For this review, take the finished solid that the model builds, in its own axes (mm). Face numbers are marked on the shaded views. A direction names the side the tool comes from. Round coordinates to 2 decimals unless told otherwise and drop trailing zeros. Write each loop counter-clockwise with the first axis right and the second up, starting at its lowest first coordinate (ties: lowest second). Pieces come first, ordered by that corner, then holes. Notation, with made-up numbers: M 69.25,70.5 L 79.25,70.5 A30 cw 79.25,93.5 Z; hole C 85,72 d3. An arc over 180 degrees is marked long. One line per question, with ' | ' between items.
```python
from build123d import *

# Parameters (mm, degrees)
SKETCH1_R               = 11
SKETCH1_R_2             = 2.669858215
BOSS_EXTRUDE1_DEPTH     = 2
SKETCH2_R               = 4.05
BOSS_EXTRUDE2_DEPTH     = 3
SKETCH3_R               = 4
SKETCH3_R_2             = 2.669858215
BOSS_EXTRUDE3_DEPTH     = 1
CHAMFER1_SIZE           = 0.6
M2_TAPPED_HOLE1_D       = 1.6
M2_5_TAPPED_HOLE1_D     = 2.05
M2_5_TAPPED_HOLE1_DEPTH = 6.35
M2_5_TAPPED_HOLE1_TIP   = 0.615882135


with BuildPart() as part:
    # Sketch1 → Boss-Extrude1 (new body)
    with BuildSketch(Plane.XY):
        Circle(SKETCH1_R)
        Circle(SKETCH1_R_2, mode=Mode.SUBTRACT)
    extrude(amount=BOSS_EXTRUDE1_DEPTH)

    # Sketch2 → Boss-Extrude2 (add)
    with BuildSketch(Plane.XY.offset(2)):
        Circle(SKETCH2_R)
    extrude(amount=BOSS_EXTRUDE2_DEPTH)

    # Sketch3 → Boss-Extrude3 (add)
    with BuildSketch(Plane(origin=(0, 0, 0), x_dir=(-1, 0, 0), z_dir=(0, 0, -1))):
        Circle(SKETCH3_R)
        Circle(SKETCH3_R_2, mode=Mode.SUBTRACT)
    extrude(amount=BOSS_EXTRUDE3_DEPTH)

    # Chamfer1
    chamfer1_edges = [part.edges().sort_by_distance(p)[0] for p in [
        (4, 0, -1),
    ]]
    chamfer(chamfer1_edges, length=CHAMFER1_SIZE)

    # M2 Tapped Hole1 (through all)
    with Locations(Plane.XY.offset(2)):
        with Locations((2.286188648, 7.666377336), (7.037526898, 3.804367906), (7.666377336, -2.286188648), (3.804367906, -7.037526898), (-2.286188648, -7.666377336), (-7.037526898, -3.804367906), (-7.666377336, 2.286188648), (-3.804367906, 7.037526898)):
            Hole(M2_TAPPED_HOLE1_D / 2)

    # M2.5 Tapped Hole1
    with Locations(Plane.XY.offset(5)):
        with Locations((0, 0)):
            Hole(M2_5_TAPPED_HOLE1_D / 2, depth=M2_5_TAPPED_HOLE1_DEPTH)
            with Locations((0, 0, -(M2_5_TAPPED_HOLE1_DEPTH + M2_5_TAPPED_HOLE1_TIP / 2))):  # 118° drill point
                Cone(0, M2_5_TAPPED_HOLE1_D / 2, M2_5_TAPPED_HOLE1_TIP, mode=Mode.SUBTRACT)


solid = part.part
```
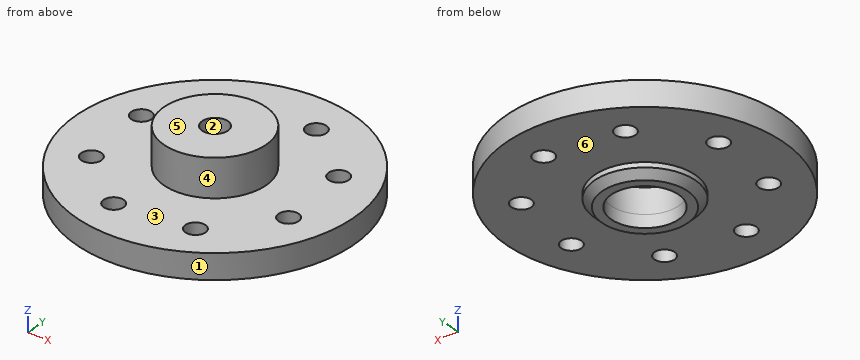
Item 1: Machinability: for the marked faces 4, 5 and 6, which of the approach directions +Z, -Z, +X, -X, +Y, -Y give a long, thin tool a straight path to every point of the face, cutting with its end or side? Answer none if there is none.
Results:
face 4: +Z | face 5: +Z, +X, -X, +Y, -Y | face 6: -Z
Item 2: Take a section at C-C (z = 1.4). State how many separate pieces and enclosed holes the cut face has, then the cut area to 3 significant figures.
Results:
separate pieces: 1 | enclosed holes: 9 | area: 342 mm2
Item 3: To check wall thickness, follow line 1 along Y through (x, z) = (1.75, 1.9); line 2 along Y through (x, z) = (0, 4.35) (3 decimals); line 3 along Z through (x, y) = (0, 7.5). State the ranges of each line that lie inside material, in increasing order. Write a range as from..to.
Results:
line 1: -10.86..-2.02, 2.02..7.07, 8.26..10.86 | line 2: -4.05..-1.025, 1.025..4.05 | line 3: 0..2
Item 4: Insertion check: pin 1 Ø5 at (x, y) = (0, 0) entering from -Z; pin 2 Ø1.8 at (x, y) = (-3.8, 7.04) entering from +Z; pin 3 Ø1.3 at (x, y) = (-2.29, -7.67) entering from +Z; pin 4 Ø1.5 at (y, z) = (-7, 1) entering from -X. Each pin has a flat end and moves straight along its axis. Give the tip position at first contact, or say it passes through.
Results:
pin 1: z = 2 | pin 2: z = 2 | pin 3: through | pin 4: x = -9.05
Item 5: Take a section at A-A (x = 0). Write out the cut boundary in (y, z) (3 decimals).
Results:
outline: M -11,0 L -4,0 L -4,-0.4 L -3.4,-1 L -2.67,-1 L -2.67,2 L -1.025,2 L -1.025,5 L -4.05,5 L -4.05,2 L -11,2 Z; M 1.025,2 L 2.67,2 L 2.67,-1 L 3.4,-1 L 4,-0.4 L 4,0 L 11,0 L 11,2 L 4.05,2 L 4.05,5 L 1.025,5 Z
Item 6: Mouldability with a two-part tool opening along X and no side actions: class the marked faces 1, 2 and 3 as +X half, -X half, draft (parallel to the pull), parting line (faces both ways), or undercut.
Results:
face 1: parting line | face 2: undercut | face 3: draft
Item 7: Take a section at D-D (z = 3.35). Write out the cut boundary in (x, y) (3 decimals), then the cut area to 3 significant figures.
Results:
outline: C 0,0 d8.1; hole C 0,0 d2.05 | area: 48.2 mm2
